Check sheet for the modelled part. Datum: model origin and axes. Units: mm. Face numbers are marked on the shaded views. A direction names the side the tool comes from. Round coordinates to 2 decimals unless told otherwise and drop trailing zeros. Loops run counter-clockwise (first coordinate to the right, second up) from the corner with the lowest first, then second, coordinate; pieces in that order, holes last. Notation, with made-up numbers: (3, 38.25) -> (59, 38.25) arc R25 cw to (59, 58.25) -> close; hole circle Ø11 at (-13.5, 5). An arc over 180 degrees is marked (long way). Return JSON: item names as keys, results as strings.
from build123d import *

# Parameters (mm, degrees)
EXTRUDE_THIN1_DEPTH     = 243.6368
CUT_EXTRUDE1_DEPTH      = 251.169323288
CUT_EXTRUDE1_DEPTH_BACK = 251.169323288
SKETCH4_R               = 14.3129


with BuildPart() as part:
    # Sketch1 → Extrude-Thin1 (new body)
    with BuildSketch(Plane(origin=(0, 0, 0), x_dir=(0, 0, -1), z_dir=(1, 0, 0))):
        with BuildLine():
            Line((-48.26, 25.4), (-2.54, 25.4))
            ThreePointArc((-2.54, 25.4), (-0.743948776, 24.656051224), (0, 22.86))
            Line((0, 22.86), (0, 2.54))
            ThreePointArc((0, 2.54), (-0.743948776, 0.743948776), (-2.54, 0))
            Line((-2.54, 0), (-48.26, 0))
            ThreePointArc((-48.26, 0), (-50.056051224, 0.743948776), (-50.8, 2.54))
            Line((-50.8, 2.54), (-50.8, 22.86))
            ThreePointArc((-50.8, 22.86), (-50.056051224, 24.656051224), (-48.26, 25.4))
        make_face()
        with BuildLine():
            Line((-48.26, 23.8125), (-2.54, 23.8125))
            ThreePointArc((-2.54, 23.8125), (-1.866480791, 23.533519209), (-1.5875, 22.86))
            Line((-1.5875, 22.86), (-1.5875, 2.54))
            ThreePointArc((-1.5875, 2.54), (-1.866480791, 1.866480791), (-2.54, 1.5875))
            Line((-2.54, 1.5875), (-48.26, 1.5875))
            ThreePointArc((-48.26, 1.5875), (-48.933519209, 1.866480791), (-49.2125, 2.54))
            Line((-49.2125, 2.54), (-49.2125, 22.86))
            ThreePointArc((-49.2125, 22.86), (-48.933519209, 23.533519209), (-48.26, 23.8125))
        make_face(mode=Mode.SUBTRACT)
    extrude(amount=-EXTRUDE_THIN1_DEPTH)

    # Sketch4 → Cut-Extrude1 (cut, two sides: drawn at the far end of the back side and taken through both)
    with BuildSketch(Plane(origin=(0, 25.4, 0), x_dir=(1, 0, 0), z_dir=(0, 1, 0)).offset(-CUT_EXTRUDE1_DEPTH_BACK)):
        with Locations(Location((-20.6629, -25.4, 0), (0, 0, 270))):
            Circle(SKETCH4_R)
        Polygon((-216.779817555, 0), (-212.369153842, -25.014116927), (-243.6368, -30.527446567), (-243.6368, 0), align=None)
    extrude(amount=CUT_EXTRUDE1_DEPTH + CUT_EXTRUDE1_DEPTH_BACK, mode=Mode.SUBTRACT)


solid = part.part
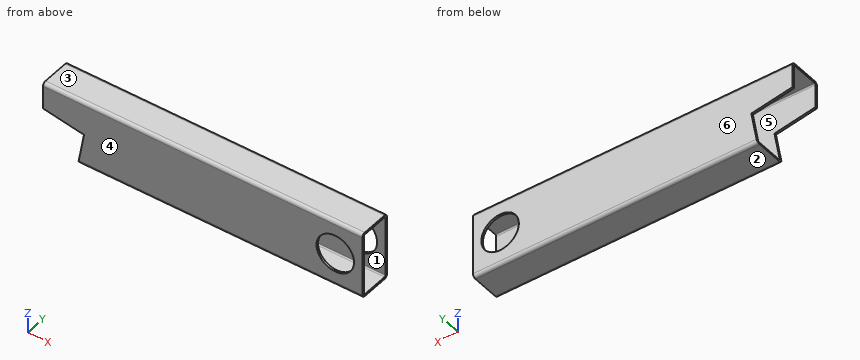
Q1. Tool access check on the marked faces 1 and 2. Record the directions out of +Z, -Z, +X, -X, +Y, -Y that give a thin tool (end or side, any length) a straight path to the whole face; none if there is none.
Results list:
{"face 1": "+X, -X", "face 2": "-Z, +X, -X, +Y, -Y"}
Q2. Section check B-B (z = 13.5). Record the boundary of the cut face in (x, y).
Results list:
{"outline": "(-214.4, 0) -> (-28.62, 0) -> (-28.62, 1.59) -> (-214.4, 1.59) -> close; (-214.4, 23.81) -> (-28.62, 23.81) -> (-28.62, 25.4) -> (-214.4, 25.4) -> close; (-12.71, 0) -> (0, 0) -> (0, 1.59) -> (-12.71, 1.59) -> close; (-12.71, 23.81) -> (0, 23.81) -> (0, 25.4) -> (-12.71, 25.4) -> close"}
Q3. Material ranges on line 1 (Y direction, x = -102.5, z = 22.5); line 2 (Z direction, x = -61, y = 5.25); line 3 (Z direction, x = -227.5, y = 15.75), recorded low to high.
Results list:
{"line 1": "0 to 1.59, 23.81 to 25.4", "line 2": "0 to 1.59, 49.21 to 50.8", "line 3": "49.21 to 50.8"}
Q4. Section check D-D (x = -221). Record the boundary of the cut face in (y, z) (1 decimal), then the cut area to 3 significant figures.
Results list:
{"outline": "(0, 26.5) -> (1.6, 26.5) -> (1.6, 48.3) arc R1 cw to (2.5, 49.2) -> (22.9, 49.2) arc R1 cw to (23.8, 48.3) -> (23.8, 26.5) -> (25.4, 26.5) -> (25.4, 48.3) arc R2.5 ccw to (22.9, 50.8) -> (2.5, 50.8) arc R2.5 ccw to (0, 48.3) -> close", "area": "110 mm^2"}
Q5. Go/stop test with a flat-tipped pin: pin 1 (12 mm diameter, centred on y = 16, z = 29.5, fed in from +X). Record where the tip stops, or that it passes through.
Results list:
{"pin 1": "through"}
Q6. Section check C-C (x = -113.5). Record the boundary of the cut face in (y, z) (1 decimal).
Results list:
{"outline": "(0, 2.5) arc R2.5 ccw to (2.5, 0) -> (22.9, 0) arc R2.5 ccw to (25.4, 2.5) -> (25.4, 48.3) arc R2.5 ccw to (22.9, 50.8) -> (2.5, 50.8) arc R2.5 ccw to (0, 48.3) -> close; hole (1.6, 2.5) arc R1 ccw to (2.5, 1.6) -> (22.9, 1.6) arc R1 ccw to (23.8, 2.5) -> (23.8, 48.3) arc R1 ccw to (22.9, 49.2) -> (2.5, 49.2) arc R1 ccw to (1.6, 48.3) -> close"}
Q7. Section check A-A (y = 10.75). Record the boundary of the cut face in (x, z).
Results list:
{"outline": "(-243.64, 49.21) -> (0, 49.21) -> (0, 50.8) -> (-243.64, 50.8) -> close; (-216.78, 0) -> (0, 0) -> (0, 1.59) -> (-216.5, 1.59) -> close"}
Q8. Draft check along Y on the marked faces 3, 4, 5 and 6. Enter one of: released by +Y, released by -Y, zero draft, split by the parting line, or undercut.
Results list:
{"face 3": "zero draft", "face 4": "released by -Y", "face 5": "undercut", "face 6": "released by +Y"}
